The model under review builds one solid part; all positions refer to its coordinate system, in mm. Face numbers are marked on the shaded views. Coordinates: 2 decimals unless noted, no trailing zeros. Answer in a Markdown table with one row per item.
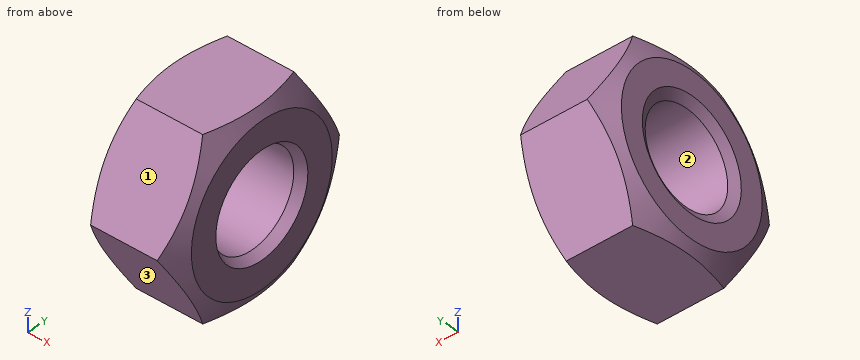
```python
from build123d import *
from OCP.BRepFilletAPI import BRepFilletAPI_MakeChamfer

# Parameters (mm, degrees)
BODY_DEPTH     = 6.8
THREAD_D       = 6.8
CHAMFER3_SIZE  = 0.676582347
CHAMFER3_SIZE2 = 0.390625


with BuildPart() as part:
    # Sketch1 → Body (new body)
    with BuildSketch(Plane.YZ):
        Polygon((-7.505553499, 0), (-3.75277675, 6.5), (3.75277675, 6.5), (7.505553499, 0), (3.75277675, -6.5), (-3.75277675, -6.5), align=None)
    extrude(amount=BODY_DEPTH)

    # Sketch2 → Chamfer1 (revolve, cut)
    with BuildSketch(Plane.XY, mode=Mode.PRIVATE) as chamfer1_sk:
        Polygon((0, 5.8), (0.984701772, 7.505553499), (0, 7.505553499), align=None)
        Polygon((6.8, 5.8), (6.8, 7.505553499), (5.815298228, 7.505553499), align=None)
    revolve(chamfer1_sk.sketch.rotate(Axis((-1.36, 0, 0), (1, 0, 0)), 299.999999999), axis=Axis((-1.36, 0, 0), (1, 0, 0)), mode=Mode.SUBTRACT)

    # Thread (through all)
    with Locations(Plane(origin=(6.8, 0, 0), x_dir=(0, 0, -1), z_dir=(1, 0, 0))):
        with Locations((0, 0)):
            Hole(THREAD_D / 2)

    # Chamfer3: one chamfer whose edges measure the first distance from different faces: ONE call of the kernel's chamfer builder (chamfer() names one face for all edges)
    chamfer3_edges_1 = [part.edges().sort_by_distance(p)[0] for p in [
        (6.8, 0, -3.4),
    ]]
    chamfer3_side_1 = [part.faces().sort_by_distance(p)[0] for p in [
        (3.4, 0, -3.4),
    ]]
    chamfer3_edges_2 = [part.edges().sort_by_distance(p)[0] for p in [
        (0, 0, -3.4),
    ]]
    chamfer3_side_2 = [part.faces().sort_by_distance(p)[0] for p in [
        (0, -2.817975613, 4.880876937),
    ]]
    chamfer3 = BRepFilletAPI_MakeChamfer(part.part.solid().wrapped)
    for e in chamfer3_edges_1:
        chamfer3.Add(CHAMFER3_SIZE, CHAMFER3_SIZE2, e.wrapped, chamfer3_side_1[0].wrapped)  # the first distance lies on this face
    for e in chamfer3_edges_2:
        chamfer3.Add(CHAMFER3_SIZE, CHAMFER3_SIZE2, e.wrapped, chamfer3_side_2[0].wrapped)  # the first distance lies on this face
    add(Compound.cast(chamfer3.Shape()), mode=Mode.REPLACE)


solid = part.part
```
Item 1: To check wall thickness, follow line 1 (Y direction, x = 0.5, z = -0.25); line 2 (Z direction, x = 3.75, y = 1.5); line 3 (Z direction, x = 2, y = 1). State the ranges of each line that lie inside material, in increasing order. Write a range as from..to.
Check values:
| item | result |
|---|---|
| line 1 | -6.66..-3.39, 3.39..6.66 |
| line 2 | -6.5..-3.05, 3.05..6.5 |
| line 3 | -6.5..-3.25, 3.25..6.5 |
Item 2: Mouldability with a two-part tool opening along Z and no side actions: class the marked faces 1, 2 and 3 as +Z half, -Z half, draft (parallel to the pull), parting line (faces both ways), or undercut.
Check values:
| item | result |
|---|---|
| face 1 | +Z half |
| face 2 | undercut |
| face 3 | -Z half |
Item 3: Clearance check with a flat-ended pin moving along its axis: pin 1 Ø1 at (x, z) = (1.5, -2.5) entering from +Y. State where the tip first meets the part, or that it passes through.
Check values:
| item | result |
|---|---|
| pin 1 | y = 6.35 |
